For this review, take the finished solid that the model builds, in its own axes (mm). Face numbers are marked on the shaded views. A direction names the side the tool comes from. Give positions to 0.01 mm unless a question says otherwise; leave off trailing zeros. Loops run counter-clockwise (first coordinate to the right, second up) from the corner with the lowest first, then second, coordinate; pieces in that order, holes last. Notation, with made-up numbers: (16, -6.5) - (32, -6.5) arc R24 cw to (32, 29.5) - close; hole circle Ø7 at (-23, 28.25). An arc over 180 degrees is marked (long way). Put each result on its own line as item: value.
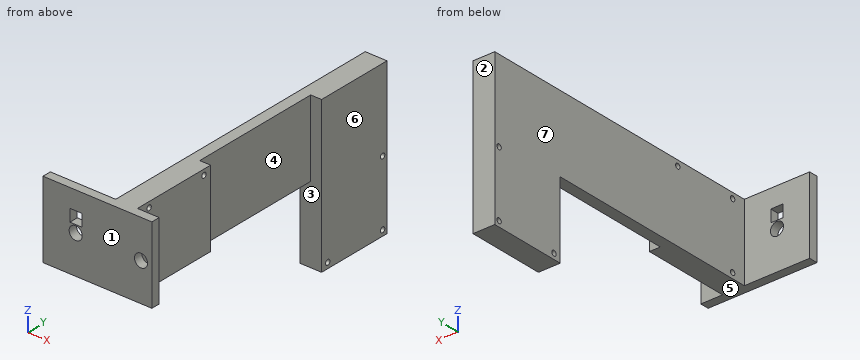
from build123d import *

# Parameters (mm, degrees)
SKETCH1_W                      = 12.7
SKETCH1_H                      = 44.45
HEIGHT_EXTRUDE_DEPTH           = 172.72
SKETCH2_R                      = 1.5
BOTTOM_FAN_MOUNT_CUTS_DEPTH    = 13.7
SKETCH3_W                      = 63.5
SKETCH3_H                      = 44.45
MOUNTING_BASE_EXTRUDE_DEPTH    = 5.08
SKETCH4_R                      = 3.81
MOUNTING_BOLT_HOLE_CUT_DEPTH   = 5.08
SKETCH6_W                      = 6.998886625
SKETCH6_H                      = 7.121323501
OPTIONAL_WIRE_ESCAPE_CUT_DEPTH = 5.08
SKETCH7_W                      = 12.7
SKETCH7_H                      = 45.266682412
BOSS_EXTRUDE1_DEPTH            = 44.45
SKETCH5_R                      = 1.5
TOP_FAN_MOUNT_CUTS_DEPTH       = 51.8
SKETCH8_W                      = 44.45
SKETCH8_H                      = 76.812549829
FILAMENT_NO_STICK_CUT_DEPTH    = 6.35


with BuildPart() as part:
    # Sketch1 → Height extrude (new body)
    with BuildSketch(Plane(origin=(0, 0, 0), x_dir=(1, 0, 0), z_dir=(0, 1, 0))):
        Rectangle(SKETCH1_W, SKETCH1_H)
    extrude(amount=HEIGHT_EXTRUDE_DEPTH)

    # Sketch2 → Bottom Fan Mount Cuts (cut, through all)
    with BuildSketch(Plane(origin=(6.35, 0, 0), x_dir=(0, 0, -1), z_dir=(1, 0, 0))):
        with Locations((-19.0000001, 8.079994)):
            Circle(SKETCH2_R)
        with Locations((19, 8.079994)):
            Circle(SKETCH2_R)
        with Locations((-19.0000001, 46.079994)):
            Circle(SKETCH2_R)
    extrude(amount=-BOTTOM_FAN_MOUNT_CUTS_DEPTH, mode=Mode.SUBTRACT)

    # Sketch3 → Mounting Base Extrude (add)
    with BuildSketch(Plane.XZ):
        with Locations((-12.7, 0)):
            Rectangle(SKETCH3_W, SKETCH3_H)
    extrude(amount=MOUNTING_BASE_EXTRUDE_DEPTH)

    # Sketch4 → Mounting Bolt Hole Cut (cut)
    with BuildSketch(Plane(origin=(0, 0, 0), x_dir=(1, 0, 0), z_dir=(0, 1, 0))):
        with Locations((12.7, 0)):
            Circle(SKETCH4_R)
        with Locations((-25.4, 0)):
            Circle(SKETCH4_R)
    extrude(amount=-MOUNTING_BOLT_HOLE_CUT_DEPTH, mode=Mode.SUBTRACT)

    # Sketch6 → Optional Wire Escape Cut (cut)
    with BuildSketch(Plane(origin=(0, 0, 0), x_dir=(1, 0, 0), z_dir=(0, 1, 0))):
        with Locations((-25.259836811, -7.950336846)):
            Rectangle(SKETCH6_W, SKETCH6_H)
    extrude(amount=-OPTIONAL_WIRE_ESCAPE_CUT_DEPTH, mode=Mode.SUBTRACT)

    # Sketch7 → Boss-Extrude1 (add)
    with BuildSketch(Plane(origin=(0, 0, -22.225), x_dir=(-1, 0, 0), z_dir=(0, 0, -1))):
        with Locations((0, 150.086658794)):
            Rectangle(SKETCH7_W, SKETCH7_H)
    extrude(amount=BOSS_EXTRUDE1_DEPTH)

    # Sketch5 → Top Fan Mount Cuts (cut, through all)
    with BuildSketch(Plane(origin=(6.35, 0, 0), x_dir=(0, 0, -1), z_dir=(1, 0, 0))):
        with Locations((25.4, 169.72)):
            Circle(SKETCH5_R)
        with Locations((63.4, 169.72)):
            Circle(SKETCH5_R)
        with Locations((63.4, 131.72)):
            Circle(SKETCH5_R)
    extrude(amount=-TOP_FAN_MOUNT_CUTS_DEPTH, mode=Mode.SUBTRACT)

    # Sketch8 → Filament no stick cut (cut)
    with BuildSketch(Plane(origin=(6.35, 0, 0), x_dir=(0, 0, -1), z_dir=(1, 0, 0))):
        with Locations((0, 89.047042674)):
            Rectangle(SKETCH8_W, SKETCH8_H)
    extrude(amount=-FILAMENT_NO_STICK_CUT_DEPTH, mode=Mode.SUBTRACT)


solid = part.part
1) Draft analysis for pull direction Y (two halves, no side actions). For the marked faces 1, 2, 3 and 4, state which applies: pulls with the +Y half, pulls with the -Y half, needs draft (parallel to the pull), parting line crosses it, or undercut.
Geometry check:
face 1: pulls with the -Y half
face 2: pulls with the +Y half
face 3: undercut
face 4: undercut
2) Take a section at B-B on x = -25.4. State the section outline as (y, z) points (3 decimals).
Geometry check:
outline: (-5.08, -22.225) - (0, -22.225) - (0, -3.81) - (-5.08, -3.81) - close; (-5.08, 3.81) - (0, 3.81) - (0, 4.39) - (-5.08, 4.39) - close; (-5.08, 11.511) - (0, 11.511) - (0, 22.225) - (-5.08, 22.225) - close
3) Insertion check: pin 1 Ø5 at (y, z) = (46.08, 19) entering from +X; pin 2 Ø8 at (x, y) = (-0.5, 66.5) entering from -Z (3 decimals); pin 3 Ø6.5 at (x, z) = (13, 10.5) entering from +Y. Each pin has a flat end and moves straight along its axis. Give the tip position at first contact, or say it passes through.
Geometry check:
pin 1: stops at x = 6.35
pin 2: stops at z = -22.225
pin 3: stops at y = 0
4) Take a section at D-D on z = -12.5. State the section outline as (x, y) points.
Geometry check:
outline: (-44.45, -5.08) - (19.05, -5.08) - (19.05, 0) - (6.35, 0) - (6.35, 50.64) - (0, 50.64) - (0, 127.45) - (6.35, 127.45) - (6.35, 172.72) - (-6.35, 172.72) - (-6.35, 0) - (-44.45, 0) - close
5) Take a section at C-C on z = 0. State the section outline as (x, y) points, and give its area (3 significant figures).
Geometry check:
outline: (-44.45, -5.08) - (-29.21, -5.08) - (-29.21, 0) - (-44.45, 0) - close; (-21.59, -5.08) - (8.89, -5.08) - (8.89, 0) - (6.35, 0) - (6.35, 50.64) - (0, 50.64) - (0, 127.45) - (6.35, 127.45) - (6.35, 172.72) - (-6.35, 172.72) - (-6.35, 0) - (-21.59, 0) - close; (16.51, -5.08) - (19.05, -5.08) - (19.05, 0) - (16.51, 0) - close
area: 1,950 mm²
6) Take a section at A-A on x = 12.7. State the section outline as (y, z) points (3 decimals).
Geometry check:
outline: (-5.08, -22.225) - (0, -22.225) - (0, -3.81) - (-5.08, -3.81) - close; (-5.08, 3.81) - (0, 3.81) - (0, 22.225) - (-5.08, 22.225) - close
7) Wall thickness on line 1 (Y direction, x = 2, z = -19); line 2 (X direction, y = -3.55, z = 0); line 3 (Y direction, x = 3.25, z = 19): over which ranges is each line inside the solid? List them lowest first.
Geometry check:
line 1: y = -5.08 to 6.58, 9.58 to 50.64, 127.45 to 172.72
line 2: x = -44.45 to -29.21, -21.59 to 8.89, 16.51 to 19.05
line 3: y = -5.08 to 6.58, 9.58 to 44.58, 47.58 to 50.64, 127.45 to 172.72
8) For the marked faces 5, 6 and 7, list the 3-axis set-ups (+Z, -Z, +X, -X, +Y, -Y) from which the entire face can be reached by the end or side of a thin tool; tool diameter is ignored.
Geometry check:
face 5: -Z, +X, -X, -Y
face 6: +Z, -Z, +X, +Y
face 7: +Z, -Z, -X, +Y
